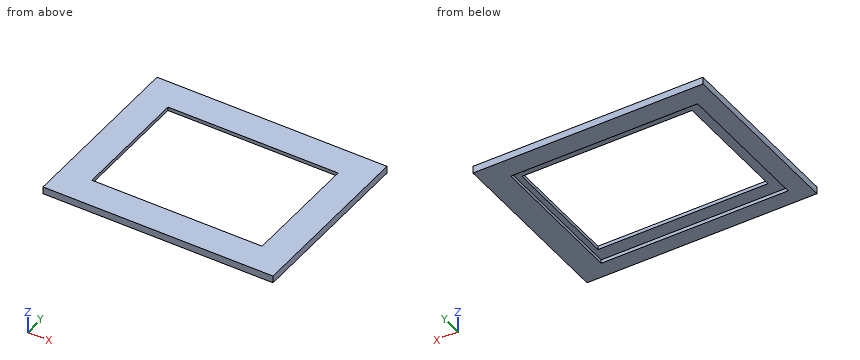
from build123d import *

# Parameters (mm, degrees)
SKETCH_W     = 192
SKETCH_H     = 150
SKETCH_W_2   = 142
SKETCH_H_2   = 100
PAD_DEPTH    = 6
SKETCH001_W  = 156
SKETCH001_H  = 119
POCKET_DEPTH = 3


with BuildPart() as part:
    # Sketch → Pad (new body)
    with BuildSketch(Plane.XY):
        with Locations((1.856875, 0.802246)):
            Rectangle(SKETCH_W, SKETCH_H)
        with Locations((1.856875, 0.802246)):
            Rectangle(SKETCH_W_2, SKETCH_H_2, mode=Mode.SUBTRACT)
    extrude(amount=PAD_DEPTH)

    # Sketch001 (on Face9 of Pad) → Pocket (cut)
    with BuildSketch(Plane(origin=(0, 0, 0), x_dir=(1, 0, 0), z_dir=(0, 0, -1))):
        with Locations((-0.66, 1)):
            Rectangle(SKETCH001_W, SKETCH001_H)
    extrude(amount=-POCKET_DEPTH, mode=Mode.SUBTRACT)


solid = part.part
The model under review builds one solid part; all positions refer to its coordinate system, in mm. Give positions to 0.01 mm unless a question says otherwise; leave off trailing zeros. Loops run counter-clockwise (first coordinate to the right, second up) from the corner with the lowest first, then second, coordinate; pieces in that order, holes last. Notation, with made-up numbers: (10, 15) -> (64, 15) arc R11 ccw to (64, 32) -> close; hole circle Ø4 at (-27, 66.5). An arc over 180 degrees is marked (long way). Write each question's results on one line, items separated by ' | '.
1) Take a section at C-C, the plane z = 4.65. Give the boundary of the cut face in (x, y), plus the area to 3 significant figures.
Conclusion:
outline: (-94.14, -74.2) -> (97.86, -74.2) -> (97.86, 75.8) -> (-94.14, 75.8) -> close; hole (-69.14, -49.2) -> (72.86, -49.2) -> (72.86, 50.8) -> (-69.14, 50.8) -> close | area: 14,600 mm^2
2) Insertion check: pin 1 Ø10 at (x, y) = (44, -46) entering from -Z. The pin has a flat end and moves straight along its axis. Give the tip position at first contact, or say it passes through.
Conclusion:
pin 1: stops at z = 3
3) Take a section at A-A, the plane y = 38. Give the boundary of the cut face in (x, z), plus the area to 3 significant figures.
Conclusion:
outline: (-94.14, 0) -> (-78.66, 0) -> (-78.66, 3) -> (-69.14, 3) -> (-69.14, 6) -> (-94.14, 6) -> close; (72.86, 3) -> (77.34, 3) -> (77.34, 0) -> (97.86, 0) -> (97.86, 6) -> (72.86, 6) -> close | area: 258 mm^2
4) Take a section at D-D, the plane y = -52.5. Give the boundary of the cut face in (x, z).
Conclusion:
outline: (-94.14, 0) -> (-78.66, 0) -> (-78.66, 3) -> (77.34, 3) -> (77.34, 0) -> (97.86, 0) -> (97.86, 6) -> (-94.14, 6) -> close
5) For line 1 along X through (y, z) = (-8.5, 4.05); line 2 along Y through (x, z) = (42, 4.4); line 3 along Y through (x, z) = (35.5, 2.65), list the stretches that pass through material, from the lowest coordinate up. Write a range as from..to.
Conclusion:
line 1: x = -94.14..-69.14, 72.86..97.86 | line 2: y = -74.2..-49.2, 50.8..75.8 | line 3: y = -74.2..-60.5, 58.5..75.8
6) Take a section at B-B, the plane x = 62. Give the boundary of the cut face in (y, z), plus the area to 3 significant figures.
Conclusion:
outline: (-74.2, 0) -> (-60.5, 0) -> (-60.5, 3) -> (-49.2, 3) -> (-49.2, 6) -> (-74.2, 6) -> close; (50.8, 3) -> (58.5, 3) -> (58.5, 0) -> (75.8, 0) -> (75.8, 6) -> (50.8, 6) -> close | area: 243 mm^2
